Can you work these out from the model? Positions are in its coordinate system, mm. Face numbers are marked on the shaded views. A direction names the side the tool comes from. Coordinates: 2 decimals unless noted, no trailing zeros. Order: outer loops, then holes, each group sorted by start corner. A loop starts at its lowest first (then second) coordinate and runs counter-clockwise, first axis right, second up. Notation, with made-up numbers: (53, 49.5) -> (95, 49.5) arc R30 cw to (95, 82.5) -> close; hole circle Ø7 at (11, -25.5). An arc over 180 degrees is marked (long way). Use a Markdown table: item, result. Add a question column.
1. Suppose I cut it at B-B, the plane x = 31. List the corners of the cut face in (y, z) for me, then the cut area to 3 significant figures.
2. For pin 1 Ø8 at (x, y) = (76.5, 62.5) entering from +Z; pin 2 Ø3.5 at (x, y) = (51.5, 24.5) entering from +Z; pin 3 Ø5 at (y, z) = (21, 5.5) entering from -X, each with a flat end and sliding along its axis, tell me the tip position at first contact or that it passes through.
3. For the marked faces 1, 2, 3, 4 and 5, which set-ups out of +Z, -Z, +X, -X, +Y, -Y let a thin tool reach every point of the face, with its end or its side?
4. Suppose I cut it at C-C, the plane y = 31.5. List the corners of the cut face in (x, z) for me, then the cut area to 3 significant figures.
5. We'd pull the mould along X, two halves only. Please class the marked faces 6, 7 and 8: pulls with the +X half, pulls with the -X half, needs draft (parallel to the pull), parting line crosses it, or undercut.
6. If I drill on line 1 along Y through (x, z) = (93.5, 5); line 2 along X through (y, z) = (26, 2.25); line 3 along X through (y, z) = (72, 5.5), over which ranges is the centre line in solid material (lowest first)? Write a range as from..to.
7. Suppose I cut it at A-A, the plane z = 12.5. List the corners of the cut face in (x, y) for me.
8. Suppose I cut it at D-D, the plane x = 48.5. List the corners of the cut face in (y, z) for me, then the cut area to 3 significant figures.
```python
from build123d import *

# Parameters (mm, degrees)
F0_W      = 85.4666158557
F0_H      = 56.3820376992
F1_DEPTH  = 1.5
F2_R      = 3
F3_W      = 51.0251373053
F3_H      = 5.0469487906
F4_DEPTH  = 8.5
F5_W      = 2.0034983754
F5_H      = 13.3438147604
F5_W_2    = 15.7416835427
F6_DEPTH  = 15.5
F7_DEPTH  = 13
F8_W      = 0.4854053259
F8_H      = 14.7926211357
F8_H_2    = 14.7911831737
F9_DEPTH  = 15.5
F10_W     = 14.5616829395
F10_H     = 12.1452622116
F11_DEPTH = 6
F12_W     = 6
F12_H     = 10.663215287
F13_DEPTH = 5
F14_R     = 1.75
F15_DEPTH = 2.5
F16_W     = 7.5255241245
F16_H     = 5.3236111999
F17_DEPTH = 2.6
F18_R     = 1.4
F19_DEPTH = 25


with BuildPart() as f1:
    # F0 (on Top) → F1 (new body)
    with BuildSketch(Plane.XY):
        with Locations((60.1496808231, 47.3746545613)):
            Rectangle(F0_W, F0_H)
    extrude(amount=F1_DEPTH)

    # F2
    f2_edges = [f1.edges().sort_by_distance(p)[0] for p in [
        (102.882989, 75.565673, 0.75),
        (17.416373, 75.565673, 0.75),
        (17.416373, 19.183636, 0.75),
        (102.882989, 19.183636, 0.75),
    ]]
    fillet(f2_edges, radius=F2_R)

    # F3 (on face) → F4 (join)
    with BuildSketch(Plane.XY.offset(1.5)):
        with Locations((50.2348765731, 71.8340054154)):
            Rectangle(F3_W, F3_H)
    extrude(amount=F4_DEPTH)

    # F5 (on face) → F6 (join)
    with BuildSketch(Plane.XY.offset(1.5)):
        with Locations((103.8847379386, 48.2480246574)):
            Rectangle(F5_W, F5_H)
        with Locations((95.0121469796, 48.2480246574)):
            Rectangle(F5_W_2, F5_H)
        with BuildLine():
            Line((104.8864871264, 72.9445666075), (102.8589658922, 72.9445666075))
            ThreePointArc((102.8589658922, 72.9445666075), (102.8769770128, 72.7555004059), (102.8829887509, 72.5656734109))
            Line((102.8829887509, 72.5656734109), (102.8829887509, 59.670612216))
            Line((102.8829887509, 59.670612216), (104.8864871264, 59.670612216))
            Line((104.8864871264, 59.670612216), (104.8864871264, 72.9445666075))
        make_face()
        with BuildLine():
            Line((102.8589658922, 72.9445666075), (87.1413052082, 72.9445666075))
            Line((87.1413052082, 72.9445666075), (87.1413052082, 59.670612216))
            Line((87.1413052082, 59.670612216), (102.8829887509, 59.670612216))
            Line((102.8829887509, 59.670612216), (102.8829887509, 72.5656734109))
            ThreePointArc((102.8829887509, 72.5656734109), (102.8769770128, 72.7555004059), (102.8589658922, 72.9445666075))
        make_face()
    extrude(amount=F6_DEPTH)

    # F5 (on face) → F7 (join)
    with BuildSketch(Plane.XY.offset(1.5)):
        with BuildLine():
            Line((102.8829887509, 22.1836357117), (102.8829887509, 37.1904186904))
            Line((102.8829887509, 37.1904186904), (83.4540203214, 37.1904186904))
            Line((83.4540203214, 37.1904186904), (83.4540203214, 21.6917544603))
            Line((83.4540203214, 21.6917544603), (102.8423895069, 21.6917544603))
            ThreePointArc((102.8423895069, 21.6917544603), (102.8728217118, 21.9368587557), (102.8829887509, 22.1836357117))
        make_face()
        with BuildLine():
            Line((104.8864871264, 37.1904186904), (102.8829887509, 37.1904186904))
            Line((102.8829887509, 37.1904186904), (102.8829887509, 22.1836357117))
            ThreePointArc((102.8829887509, 22.1836357117), (102.8728217118, 21.9368587557), (102.8423895069, 21.6917544603))
            Line((102.8423895069, 21.6917544603), (104.8864871264, 21.6917544603))
            Line((104.8864871264, 21.6917544603), (104.8864871264, 37.1904186904))
        make_face()
    extrude(amount=F7_DEPTH)

    # F8 (on face) → F9 (join)
    with BuildSketch(Plane.XY.offset(17)):
        with Locations((104.6437844634, 66.3045793772)):
            Rectangle(F8_W, F8_H)
        with Locations((104.6437844634, 48.2392385602)):
            Rectangle(F8_W, F8_H_2)
    extrude(amount=-F9_DEPTH)

    # F10 (on face) → F11 (join)
    with BuildSketch(Plane.XY.offset(1.5)):
        with Locations((49.7219525278, 23.7262044102)):
            Rectangle(F10_W, F10_H)
    extrude(amount=F11_DEPTH)

    # F12 (on face) → F13 (join)
    with BuildSketch(Plane.XY.offset(1.5)):
        with Locations((71.8380571604, 24.5152433552)):
            Rectangle(F12_W, F12_H)
    extrude(amount=F13_DEPTH)

    # F14 (on face) → F15 (join)
    with BuildSketch(Plane.XZ.offset(-19.1836357117)):
        with BuildLine():
            ThreePointArc((71.8380571604, 6.5), (70.0702902074, 2.232233047), (74.3380571604, 4))
            ThreePointArc((74.3380571604, 4), (73.6058241133, 5.767766953), (71.8380571604, 6.5))
        make_face()
        with Locations((71.8380571604, 4)):
            Circle(F14_R, mode=Mode.SUBTRACT)
    extrude(amount=F15_DEPTH)

    # F16 (on face) → F17 (join)
    with BuildSketch(Plane.XY.offset(1.5)):
        with Locations((28.2411361113, 21.2340727448)):
            Rectangle(F16_W, F16_H)
    extrude(amount=F17_DEPTH)

    # F18 (on face) → F19 (cut)
    with BuildSketch(Plane.XY.offset(1.5)):
        with Locations((79.0960954428, 71.6403754205)):
            Circle(F18_R)
        with Locations((79.0960954428, 22.6403754205)):
            Circle(F18_R)
        with Locations((21.0960954428, 22.6403754205)):
            Circle(F18_R)
        with Locations((21.0960954428, 71.6403754205)):
            Circle(F18_R)
    extrude(amount=-F19_DEPTH, mode=Mode.SUBTRACT)


solid = f1.part
```
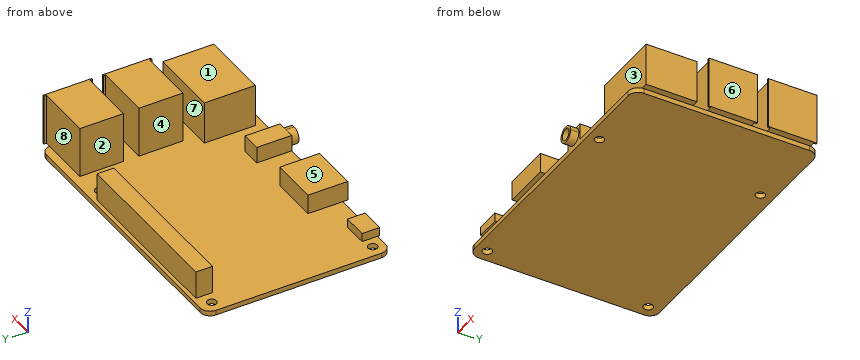
Worked out:
| question | item | result |
|---|---|---|
| 1 | outline | (18.57, 1.5) -> (19.18, 1.5) -> (19.18, 0) -> (75.57, 0) -> (75.57, 1.5) -> (74.36, 1.5) -> (74.36, 10) -> (69.31, 10) -> (69.31, 1.5) -> (23.9, 1.5) -> (23.9, 4.1) -> (18.57, 4.1) -> close |
| 1 | area | 141 mm² |
| 2 | pin 1 | stops at z = 1.5 |
| 2 | pin 2 | stops at z = 7.5 |
| 2 | pin 3 | stops at x = 24.48 |
| 3 | face 1 | +Z, +X, -X, -Y |
| 3 | face 2 | +Z, +Y |
| 3 | face 3 | +Z, +X, -Y |
| 3 | face 4 | +Z, -X, +Y |
| 3 | face 5 | +Z, -X, -Y |
| 4 | outline | (17.42, 0) -> (102.88, 0) -> (102.88, 1.5) -> (104.89, 1.5) -> (104.89, 14.5) -> (83.45, 14.5) -> (83.45, 1.5) -> (17.42, 1.5) -> close |
| 4 | area | 407 mm² |
| 5 | face 6 | pulls with the +X half |
| 5 | face 7 | needs draft |
| 5 | face 8 | undercut |
| 6 | line 1 | y = 21.69..37.19, 41.58..54.92, 59.67..72.94 |
| 6 | line 2 | x = 42.44..57, 68.84..74.84, 83.45..104.89 |
| 6 | line 3 | x = 24.72..75.75, 87.14..104.89 |
| 7 | outline | (83.45, 21.69) -> (104.89, 21.69) -> (104.89, 37.19) -> (83.45, 37.19) -> close; (87.14, 41.58) -> (104.4, 41.58) -> (104.4, 40.84) -> (104.89, 40.84) -> (104.89, 55.63) -> (104.4, 55.63) -> (104.4, 54.92) -> (87.14, 54.92) -> close; (87.14, 59.67) -> (104.4, 59.67) -> (104.4, 58.91) -> (104.89, 58.91) -> (104.89, 73.7) -> (104.4, 73.7) -> (104.4, 72.94) -> (87.14, 72.94) -> close |
| 8 | outline | (17.65, 1.5) -> (19.18, 1.5) -> (19.18, 0) -> (75.57, 0) -> (75.57, 1.5) -> (74.36, 1.5) -> (74.36, 10) -> (69.31, 10) -> (69.31, 1.5) -> (29.8, 1.5) -> (29.8, 7.5) -> (17.65, 7.5) -> close |
| 8 | area | 200 mm² |
